The drawing under review shows one solid part. Ordinate dimensions are in mm from its lowest x, y, z. A direction names the side the tool comes from. Give positions to 0.01 mm unless a question says otherwise; leave off trailing zeros. Write each loop counter-clockwise with the first axis right and the second up, starting at its lowest first coordinate (ties: lowest second). Pieces come first, ordered by that corner, then holes.
Q1. Machinability: for the marked faces 1 and 2, which of the approach directions +Z, -Z, +X, -X, +Y, -Y give a long, thin tool a straight path to every point of the face, cutting with its end or side? Answer none if there is none.
Q2. We need section A-A (z = 6). Write out the cut boundary in (x, y).
Q3. We need section C-C (y = 29). Write out the cut boundary in (x, z).
Q4. For line 1 (Y direction, x = 6.5, z = 70); line 2 (X direction, y = 23, z = 63); line 3 (Y direction, x = 65, z = 29), list the stretches that pass through material, from the lowest coordinate up.
Q5. Insertion check: P1, Ø4, axis at y = 15, z = 23, coming from the -X side; P2, Ø23, axis at y = 46.5, z = 48, coming from the +X side. Each pin has a flat end and moves straight along its axis. Give the tip position at first contact, or say it passes through.
Q6. We need section D-D (x = 46). Write out the cut boundary in (y, z).
Q7. We need section B-B (z = 38). Write out the cut boundary in (x, y).
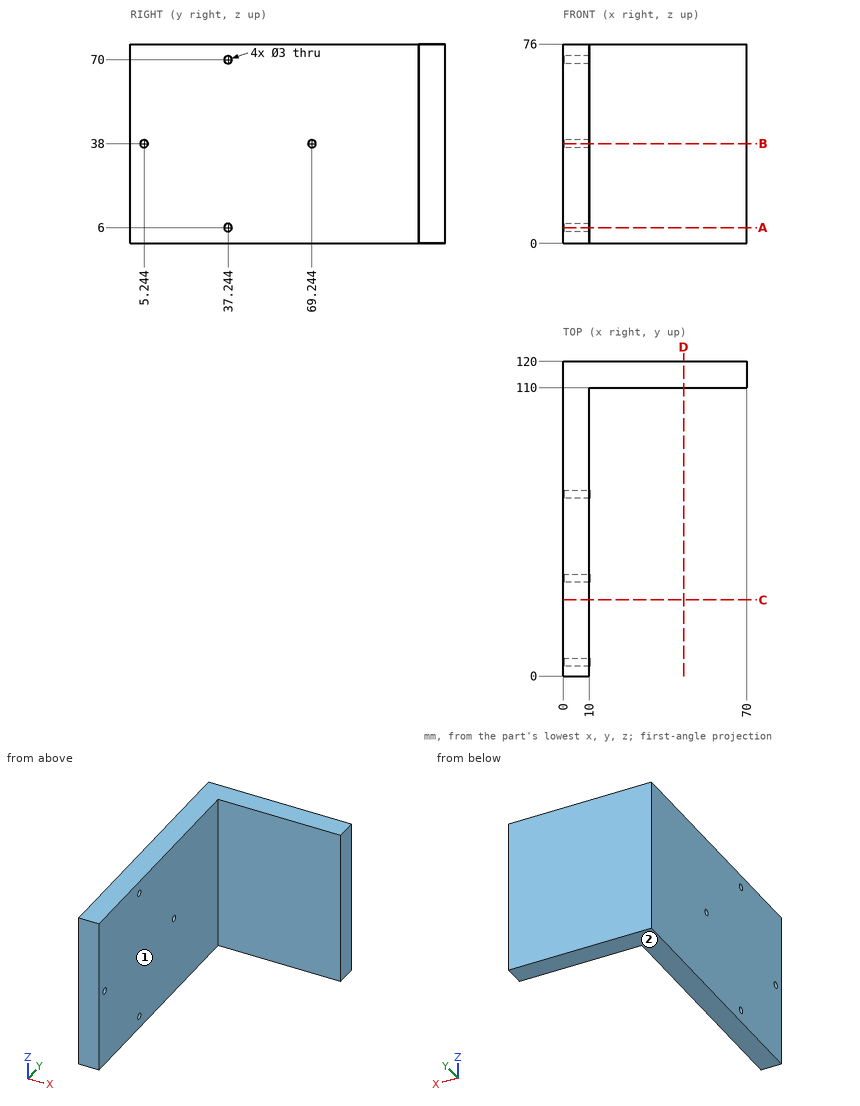
Computed:
1. face 1: +Z, -Z, +X, -Y
1. face 2: -Z, +X, -X, +Y, -Y
2. outline: (0, 0) - (10, 0) - (10, 35.74) - (0, 35.74) - close; (0, 38.74) - (10, 38.74) - (10, 110) - (70, 110) - (70, 120) - (0, 120) - close
3. outline: (0, 0) - (10, 0) - (10, 76) - (0, 76) - close
4. line 1: y = 0 to 35.74, 38.74 to 120
4. line 2: x = 0 to 10
4. line 3: y = 110 to 120
5. P1: stops at x = 0
5. P2: stops at x = 10
6. outline: (110, 0) - (120, 0) - (120, 76) - (110, 76) - close
7. outline: (0, 0) - (10, 0) - (10, 3.74) - (0, 3.74) - close; (0, 6.74) - (10, 6.74) - (10, 67.74) - (0, 67.74) - close; (0, 70.74) - (10, 70.74) - (10, 110) - (70, 110) - (70, 120) - (0, 120) - close
